```python
from build123d import *

# Parameters (mm, degrees)
SKETCH1_W           = 45.3
SKETCH1_H           = 26.1
BOSS_EXTRUDE1_DEPTH = 17.2
FILLET1_R           = 3
BOSS_EXTRUDE2_START = 4
SKETCH1_3_W         = 2.7
SKETCH1_3_H         = 19.5
BOSS_EXTRUDE2_DEPTH = 8.5


with BuildPart() as part:
    # Sketch1 → Boss-Extrude1 (new body)
    with BuildSketch(Plane(origin=(0, 0, 0), x_dir=(1, 0, 0), z_dir=(0, 1, 0))):
        with Locations((-9.556070131, 3.224117647)):
            Rectangle(SKETCH1_W, SKETCH1_H)
    extrude(amount=BOSS_EXTRUDE1_DEPTH)

    # Fillet1
    fillet1_edges = [part.edges().sort_by_distance(p)[0] for p in [
        (-9.556070131, 17.2, -16.274117647),
        (-9.556070131, 17.2, 9.825882353),
        (-9.556070131, 0, -16.274117647),
        (-9.556070131, 0, 9.825882353),
    ]]
    fillet(fillet1_edges, radius=FILLET1_R)

    # Sketch1_3 → Boss-Extrude2 (add)
    with BuildSketch(Plane(origin=(0, 0, 0), x_dir=(1, 0, 0), z_dir=(0, 1, 0)).offset(BOSS_EXTRUDE2_START)):
        with Locations((-33.556070131, 2.724117647)):
            Rectangle(SKETCH1_3_W, SKETCH1_3_H)
    extrude(amount=BOSS_EXTRUDE2_DEPTH)


solid = part.part
```
The listing builds one solid part. Answer for the finished solid, in the listing's coordinates (mm). A direction names the side the tool comes from. Coordinates: 2 decimals unless noted, no trailing zeros. Loops run counter-clockwise (first coordinate to the right, second up) from the corner with the lowest first, then second, coordinate; pieces in that order, holes last. Notation, with made-up numbers: (63.5, 73) - (108.5, 73) arc R25 cw to (108.5, 86) - close; hole circle Ø3 at (6.5, -13.5). An arc over 180 degrees is marked (long way). Use a Markdown table: item, result. Add a question column.
1) Given pin 1 (2 mm diameter, centred on x = -33.5, y = 8.5, fed in from -Z); pin 2 (3 mm diameter, centred on x = -34, y = 7, fed in from +Z); pin 3 (3 mm diameter, centred on x = -34, z = -6.5, fed in from -Y), each flat-ended and moving along its own axis, determine where each tip first touches the part or whether it passes through.
2) Find the intervals of material crossed by line 1 (X direction, y = 3.5, z = -11.5); line 2 (Y direction, x = 4, z = 7.25); line 3 (Z direction, x = 1, y = 14.5), in increasing order.
3) The part is cut by section C-C, the plane y = 1.5. Give the vertices of the cut face in (x, z), and give its area (3 significant figures).
4) The part is cut by section A-A, the plane z = -4.5. Give the vertices of the cut face in (x, y).
5) For faces 1 (the flat face through (-10, 17.2, -3)), 2 (the flat face through (-34, 12.5, -3)), 3 (the flat face through (-34, 4, -3)), 4 (the flat face through (-34, 8, 7.026)), 5 (the flat face through (-34, 8, -12.474)), determine the directions among +Z, -Z, +X, -X, +Y, -Y from which every point of the face is accessible in a straight line to the end or side of a thin tool.
6) The mould has two halves that part along Y. Classify faces 6 (the cylindrical face through (-9.24, 16.3, 8.97)), 7 (the flat face through (-32.206, 3, -3)), 8 (the flat face through (-10, 0, -3)): released by +Y, released by -Y, zero draft, split by the parting line, or undercut.
7) The part is cut by section B-B, the plane x = 3. Give the vertices of the cut face in (y, z).
8) The part is cut by section D-D, the plane z = 8.25. Give the vertices of the cut face in (x, y).
Here are the results:
| question | item | result |
|---|---|---|
| 1 | pin 1 | stops at z = -12.47 |
| 1 | pin 2 | stops at z = 7.03 |
| 1 | pin 3 | stops at y = 4 |
| 2 | line 1 | x = -32.21 to 13.09 |
| 2 | line 2 | y = 0.03 to 17.17 |
| 2 | line 3 | z = -16.26 to 9.81 |
| 3 | outline | (-32.21, -15.87) - (13.09, -15.87) - (13.09, 9.42) - (-32.21, 9.42) - close |
| 3 | area | 1,150 mm^2 |
| 4 | outline | (-34.91, 4) - (-32.21, 4) - (-32.21, 0) - (13.09, 0) - (13.09, 17.2) - (-32.21, 17.2) - (-32.21, 12.5) - (-34.91, 12.5) - close |
| 5 | face 1 | +Z, -Z, +X, -X, +Y |
| 5 | face 2 | +Z, -Z, -X, +Y |
| 5 | face 3 | +Z, -Z, -X, -Y |
| 5 | face 4 | +Z, -X, +Y, -Y |
| 5 | face 5 | -Z, -X, +Y, -Y |
| 6 | face 6 | released by +Y |
| 6 | face 7 | zero draft |
| 6 | face 8 | released by -Y |
| 7 | outline | (0, -13.27) arc R3 ccw to (3, -16.27) - (14.2, -16.27) arc R3 ccw to (17.2, -13.27) - (17.2, 6.83) arc R3 ccw to (14.2, 9.83) - (3, 9.83) arc R3 ccw to (0, 6.83) - close |
| 8 | outline | (-32.21, 0.36) - (13.09, 0.36) - (13.09, 16.84) - (-32.21, 16.84) - close |
